```python
from build123d import *

# Parameters (mm, degrees)
BOSS_EXTRUDE1_DEPTH   = 4.7625
SKETCH2_R             = 3.5
CUT_EXTRUDE1_DEPTH    = 3.2625
SKETCH3_R             = 3.125
CUT_EXTRUDE2_DEPTH    = 2.5
SKETCH6_R             = 3.125
CUT_EXTRUDE5_DEPTH    = 5.7625
SKETCH7_R             = 3.5
CUT_EXTRUDE6_DEPTH    = 3.2625
M3X0_5_TAPPED_HOLE1_D = 2.5
M3X0_5_TAPPED_HOLE2_D = 2.5


with BuildPart() as part:
    # Sketch1 → Boss-Extrude1 (new body)
    with BuildSketch(Plane(origin=(0, 0, 0), x_dir=(1, 0, 0), z_dir=(0, 1, 0))):
        with BuildLine():
            ThreePointArc((-28.349392947, 12.884852573), (-49.5, 0), (-28.349392947, -12.884852573))
            ThreePointArc((-28.349392947, -12.884852573), (0, -6), (28.349392947, -12.884852573))
            ThreePointArc((28.349392947, -12.884852573), (49.5, 0), (28.349392947, 12.884852573))
            ThreePointArc((28.349392947, 12.884852573), (0, 6), (-28.349392947, 12.884852573))
        make_face()
    extrude(amount=BOSS_EXTRUDE1_DEPTH)

    # Sketch2 → Cut-Extrude1 (cut)
    with BuildSketch(Plane(origin=(0, 4.7625, 0), x_dir=(1, 0, 0), z_dir=(0, 1, 0))):
        with Locations((-35, 0)):
            Circle(SKETCH2_R)
    extrude(amount=-CUT_EXTRUDE1_DEPTH, mode=Mode.SUBTRACT)

    # Sketch3 → Cut-Extrude2 (cut, through all)
    with BuildSketch(Plane(origin=(0, 1.5, 0), x_dir=(1, 0, 0), z_dir=(0, 1, 0))):
        with Locations((-35, 0)):
            Circle(SKETCH3_R)
    extrude(amount=-CUT_EXTRUDE2_DEPTH, mode=Mode.SUBTRACT)

    # Sketch6 → Cut-Extrude5 (cut, through all)
    with BuildSketch(Plane.XZ):
        with Locations((35, 0)):
            Circle(SKETCH6_R)
    extrude(amount=-CUT_EXTRUDE5_DEPTH, mode=Mode.SUBTRACT)

    # Sketch7 → Cut-Extrude6 (cut)
    with BuildSketch(Plane.XZ):
        with Locations((35, 0)):
            Circle(SKETCH7_R)
    extrude(amount=-CUT_EXTRUDE6_DEPTH, mode=Mode.SUBTRACT)

    # M3x0.5 Tapped Hole1 (through all)
    with Locations(Plane(origin=(0, 4.7625, 0), x_dir=(-1, 0, 0), z_dir=(0, 1, 0))):
        with Locations((30.5, 7.794228634), (44, 0), (30.5, -7.794228634)):
            Hole(M3X0_5_TAPPED_HOLE1_D / 2)

    # M3x0.5 Tapped Hole2 (through all)
    with Locations(Plane.XZ):
        with Locations((43.999848922, -0.052147689), (30.5, 7.794228634), (30.5, -7.794228634)):
            Hole(M3X0_5_TAPPED_HOLE2_D / 2)


solid = part.part
```
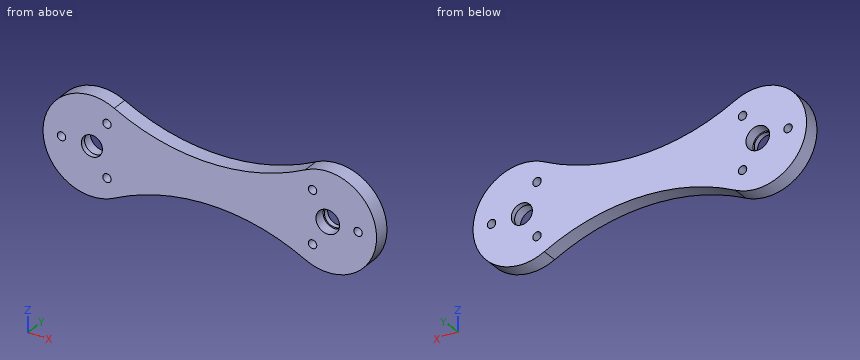
Geometry check sheet. Reference: the model listing, model coordinates, mm. Round coordinates to 2 decimals unless told otherwise and drop trailing zeros. Order: outer loops, then holes, each group sorted by start corner. A loop starts at its lowest first (then second) coordinate and runs counter-clockwise, first axis right, second up. Notation, with made-up numbers: (-27.75, -40) -> (-5.75, -40) arc R23 cw to (-5.75, -21) -> close; hole circle Ø3 at (-37, 81). An arc over 180 degrees is marked (long way). Return JSON: item names as keys, results as strings. Group by question number.
Q1. Gauge pin test, flat ends, axial feed: pin 1 (3.5 mm diameter, centred on x = 36.5, z = 0.5, fed in from -Y); pin 2 (1.5 mm diameter, centred on y = 4, z = 6.5, fed in from -X); pin 3 (6.5 mm diameter, centred on x = -35, z = 0, fed in from +Y). Record the tip position at first contact, or that the pin passes through.
Q2. Section check B-B, the plane z = 11.25. Record the boundary of the cut face in (x, y), plus the area to 3 significant figures.
Q3. Material ranges on probe 1 along X at (y, z) = (1.4, -0.5); probe 2 along X at (y, z) = (3.2, -1.75); probe 3 along X at (y, z) = (3.4, -2), recorded low to high. Write a range as from..to.
Q4. Section check C-C, the plane x = -6.5. Record the boundary of the cut face in (y, z).
Q5. Section check D-D, the plane z = -4.75. Record the boundary of the cut face in (x, y), plus the area to 3 significant figures.
Numbers:
{
 "1": {"pin 1": "y = 3.26", "pin 2": "x = -48.31", "pin 3": "y = 1.5"},
 "2": {"outline": "(-44.15, 0) -> (-24.93, 0) -> (-24.93, 4.76) -> (-44.15, 4.76) -> close; (24.93, 0) -> (44.15, 0) -> (44.15, 4.76) -> (24.93, 4.76) -> close", "area": "183 mm^2"},
 "3": {"probe 1": "-49.49..-45.15, -42.85..-38.08, -31.92..31.54, 38.46..42.83, 45.17..49.49", "probe 2": "-49.39..-38.03, -31.97..31.97, 38.03..49.39", "probe 3": "-49.36..-37.87, -32.13..32.6, 37.4..49.36"},
 "4": {"outline": "(0, -6.34) -> (4.76, -6.34) -> (4.76, 6.34) -> (0, 6.34) -> close"},
 "5": {"outline": "(-48.7, 0) -> (48.7, 0) -> (48.7, 4.76) -> (-48.7, 4.76) -> close", "area": "464 mm^2"}
}
